Build history of the part. All positions in model axes, mm. Face numbers are marked on the shaded views. A direction names the side the tool comes from. Give positions to 0.01 mm unless a question says otherwise; leave off trailing zeros. Order: outer loops, then holes, each group sorted by start corner. A loop starts at its lowest first (then second) coordinate and runs counter-clockwise, first axis right, second up. Notation, with made-up numbers: M 63,38.5 L 103,38.5 A15 ccw 103,55.5 Z; hole C -28,-23 d7. An arc over 180 degrees is marked long. One line per item, written item: value.
from build123d import *

# Parameters (mm, degrees)
F0_W     = 76.2
F0_H     = 76.2
F0_W_2   = 2.54
F0_H_2   = 59.69
F1_DEPTH = 76.2


# Not quite as in the source:
# - the program builds the solid bodies; features that only make, move or delete a surface that nothing else refers to are left out


with BuildPart() as f1:
    # F0 (on Top) → F1 (new body)
    with BuildSketch(Plane.XY):
        with Locations((-38.1, 38.1)):
            Rectangle(F0_W, F0_H)
        Polygon((-58.42, 69.85), (-17.78, 69.85), (-17.78, 67.945), (-17.78, 8.255), (-17.78, 6.35), (-58.42, 6.35), (-58.42, 8.255), (-58.42, 67.945), align=None, mode=Mode.SUBTRACT)
        with Locations((-57.15, 38.1)):
            Rectangle(F0_W_2, F0_H_2)
        with Locations((-19.05, 38.1)):
            Rectangle(F0_W_2, F0_H_2)
    extrude(amount=F1_DEPTH)


with BuildPart() as f1_1:
    # F3: moved
    add(f1.part.moved(Location((0, 106.934, 0))))


with BuildPart() as f1_2:
    # F6: moved
    add(f1_1.part.moved(Location((38.1, -144.526, 11.938))))


solid = f1_2.part
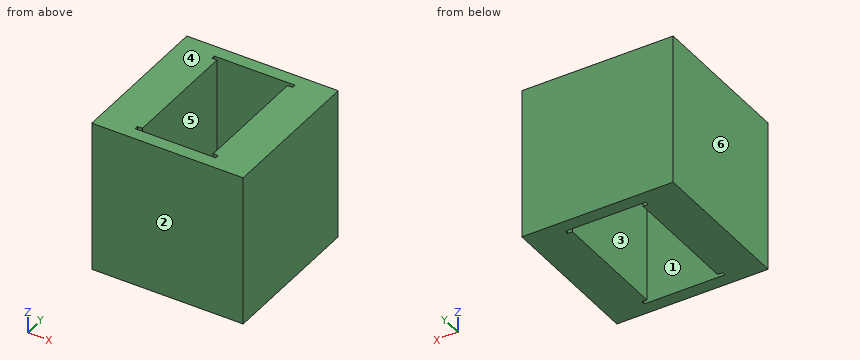
1) Saw through at C-C, the plane z = 35.5. Write the cut outline in (x, y), then the cut area to 3 significant figures.
Check values:
outline: M -38.1,-37.59 L 38.1,-37.59 L 38.1,38.61 L -38.1,38.61 Z; hole M -20.32,-31.24 L 20.32,-31.24 L 20.32,-29.34 L 17.78,-29.34 L 17.78,30.35 L 20.32,30.35 L 20.32,32.26 L -20.32,32.26 L -20.32,30.35 L -17.78,30.35 L -17.78,-29.34 L -20.32,-29.34 Z
area: 3,530 mm^2
2) Drill centre lines: probe 1 along Y at (x, z) = (-4.5, 31); probe 2 along Y at (x, z) = (-19, 67); probe 3 along X at (y, z) = (21.5, 25). Where is each one in solid material? Low to high. Write a range as from..to.
Check values:
probe 1: -37.59..-31.24, 32.26..38.61
probe 2: -37.59..-31.24, -29.34..30.35, 32.26..38.61
probe 3: -38.1..-17.78, 17.78..38.1
3) Pin check, flat tip, straight feed: pin 1 (12 mm diameter, centred on x = -10, y = 0, fed in from +Z). Stop position of the tip, or through.
Check values:
pin 1: through
4) Saw through at A-A, the plane x = 7. Write the cut outline in (y, z), then the cut area to 3 significant figures.
Check values:
outline: M -37.59,11.94 L -31.24,11.94 L -31.24,88.14 L -37.59,88.14 Z; M 32.26,11.94 L 38.61,11.94 L 38.61,88.14 L 32.26,88.14 Z
area: 968 mm^2
5) Mould opens along X. For the marked faces 3, 4, 5 and 6 say: released by +X, released by -X, zero draft, split by the parting line, or undercut.
Check values:
face 3: undercut
face 4: zero draft
face 5: undercut
face 6: released by -X
6) Tool access for the marked faces 1 and 2: list every direction of +Z, -Z, +X, -X, +Y, -Y with a clear straight run to the whole face (end or side of a thin tool).
Check values:
face 1: +Z, -Z
face 2: +Z, -Z, +X, -X, -Y
7) Saw through at B-B, the plane y = 3.5. Write the cut outline in (x, z).
Check values:
outline: M -38.1,11.94 L -17.78,11.94 L -17.78,88.14 L -38.1,88.14 Z; M 17.78,11.94 L 38.1,11.94 L 38.1,88.14 L 17.78,88.14 Z
